```python
from build123d import *

# Parameters (mm, degrees)
ESQUISSE1_W                                        = 100
ESQUISSE1_H                                        = 50
BOSS_EXTRU_1_DEPTH                                 = 10
ESQUISSE2_W                                        = 100
ESQUISSE2_H                                        = 8
BOSS_EXTRU_2_DEPTH                                 = 30
ESQUISSE3_W                                        = 10
ESQUISSE3_H                                        = 34
BOSS_EXTRU_3_DEPTH                                 = 30
ESQUISSE5_R                                        = 5.25
ENL_V_MAT_EXTRU_1_DEPTH                            = 111.566721937
ENL_V_MAT_EXTRU_4_DEPTH                            = 82.240384046
CHAMBRAGE_POUR_VIS_T_TE_RONDE_BOMB_E_M_D           = 5.5
CHAMBRAGE_POUR_VIS_T_TE_RONDE_BOMB_E_M_CBORE_D     = 10
CHAMBRAGE_POUR_VIS_T_TE_RONDE_BOMB_E_M_CBORE_DEPTH = 5


with BuildPart() as part:
    # Esquisse1 → Boss.-Extru.1 (new body)
    with BuildSketch(Plane(origin=(0, 0, 0), x_dir=(1, 0, 0), z_dir=(0, 1, 0))):
        Rectangle(ESQUISSE1_W, ESQUISSE1_H)
    extrude(amount=BOSS_EXTRU_1_DEPTH)

    # Esquisse2 → Boss.-Extru.2 (add)
    with BuildSketch(Plane(origin=(0, 10, 0), x_dir=(1, 0, 0), z_dir=(0, 1, 0))):
        with Locations((0, -21)):
            Rectangle(ESQUISSE2_W, ESQUISSE2_H)
        with Locations((0, 21)):
            Rectangle(ESQUISSE2_W, ESQUISSE2_H)
    extrude(amount=BOSS_EXTRU_2_DEPTH)

    # Esquisse3 → Boss.-Extru.3 (add)
    with BuildSketch(Plane(origin=(0, 10, 0), x_dir=(1, 0, 0), z_dir=(0, 1, 0))):
        with Locations((-45, 0)):
            Rectangle(ESQUISSE3_W, ESQUISSE3_H)
    extrude(amount=BOSS_EXTRU_3_DEPTH)

    # Esquisse5 → Enlèv. mat.-Extru.1 (cut, through all)
    with BuildSketch(Plane.ZY.offset(50)):
        with Locations((0, 25)):
            Circle(ESQUISSE5_R)
    extrude(amount=-ENL_V_MAT_EXTRU_1_DEPTH, mode=Mode.SUBTRACT)

    # Esquisse8 → Enlèv. mat.-Extru.4 (cut, through all)
    with BuildSketch(Plane.XY.offset(25)):
        with BuildLine():
            Line((-20, 28.5), (40, 28.5))
            ThreePointArc((40, 28.5), (43.5, 25), (40, 21.5))
            Line((40, 21.5), (-20, 21.5))
            ThreePointArc((-20, 21.5), (-23.5, 25), (-20, 28.5))
        make_face()
    extrude(amount=-ENL_V_MAT_EXTRU_4_DEPTH, mode=Mode.SUBTRACT)

    # Chambrage pour vis à tête ronde bombée M51 (through all)
    with Locations(Plane(origin=(0, 10, 0), x_dir=(1, 0, 0), z_dir=(0, 1, 0))):
        with Locations((-25, 0), (0, 0)):
            CounterBoreHole(CHAMBRAGE_POUR_VIS_T_TE_RONDE_BOMB_E_M_D / 2, CHAMBRAGE_POUR_VIS_T_TE_RONDE_BOMB_E_M_CBORE_D / 2, CHAMBRAGE_POUR_VIS_T_TE_RONDE_BOMB_E_M_CBORE_DEPTH)


solid = part.part
```
Input: part model. Units: mm. Frame: model coordinates. A direction names the side the tool comes from. Coordinates: 2 decimals unless noted, no trailing zeros. Loops run counter-clockwise (first coordinate to the right, second up) from the corner with the lowest first, then second, coordinate; pieces in that order, holes last. Notation, with made-up numbers: (25.5, 34.25) - (61.5, 34.25) arc R29 ccw to (61.5, 54.25) - close; hole circle Ø1 at (39, 86). An arc over 180 degrees is marked (long way). Answer in a Markdown table with one row per item.
(1) Cut plane B-B on x = 0. Output: boundary loops of the cut face in (y, z).
Model answer:
| item | result |
|---|---|
| outline | (0, -25) - (21.5, -25) - (21.5, -17) - (10, -17) - (10, -5) - (5, -5) - (5, -2.75) - (0, -2.75) - close; (0, 2.75) - (5, 2.75) - (5, 5) - (10, 5) - (10, 17) - (21.5, 17) - (21.5, 25) - (0, 25) - close; (28.5, -25) - (40, -25) - (40, -17) - (28.5, -17) - close; (28.5, 17) - (40, 17) - (40, 25) - (28.5, 25) - close |
(2) Material intervals for L1, parallel to Y at x = -45.5, z = 0; L2, parallel to Y at x = 22, z = 18; L3, parallel to Z at x = 5, y = 29.5, sorted ascending. Write a range as from..to.
Model answer:
| item | result |
|---|---|
| L1 | y = 0..19.75, 30.25..40 |
| L2 | y = 0..21.5, 28.5..40 |
| L3 | z = -25..-17, 17..25 |
(3) Set-up query: faces 5 (the face through (2.2, 5, 2.2)), 6 (the face through (4, 21, 17)), 7 (the face through (10, 28.5, -21)). Return all of +Z, -Z, +X, -X, +Y, -Y with unobstructed straight access to the full face (end or side cutting, diameter ignored); none if empty.
Model answer:
| item | result |
|---|---|
| face 5 | +Y |
| face 6 | +X, +Y |
| face 7 | +Z, -Z |
(4) Mould query, pull axis X, two halves, no side actions, for faces 1 (the face through (-45.07, 20.34, 2.42)), 2 (the face through (50, 6, 6)), 3 (the face through (-23.5, 24.9, 21.1)), 4 (the face through (10, 28.5, 21)). Classes: pulls with the +X half, pulls with the -X half, needs draft (parallel to the pull), parting line crosses it, or undercut.
Model answer:
| item | result |
|---|---|
| face 1 | needs draft |
| face 2 | pulls with the +X half |
| face 3 | undercut |
| face 4 | undercut |
(5) Cut plane C-C on y = 25. Output: boundary loops of the cut face in (x, z), plus the area to 3 significant figures.
Model answer:
| item | result |
|---|---|
| outline | (-50, -25) - (-23.5, -25) - (-23.5, -17) - (-40, -17) - (-40, -5.25) - (-50, -5.25) - close; (-50, 5.25) - (-40, 5.25) - (-40, 17) - (-23.5, 17) - (-23.5, 25) - (-50, 25) - close; (43.5, -25) - (50, -25) - (50, -17) - (43.5, -17) - close; (43.5, 17) - (50, 17) - (50, 25) - (43.5, 25) - close |
| area | 763 mm² |
(6) Pin query (flat end, axial travel): P1, Ø9, axis at x = 14, z = 20.5, coming from the -Y side; P2, Ø11, axis at x = -1, z = 2.5, coming from the +Y side; P3, Ø6, axis at x = -25, z = 0, coming from the +Y side. Return the tip coordinate at first contact, or that it passes through.
Model answer:
| item | result |
|---|---|
| P1 | stops at y = 0 |
| P2 | stops at y = 10 |
| P3 | stops at y = 5 |
(7) Cut plane D-D on x = 21. Output: boundary loops of the cut face in (y, z).
Model answer:
| item | result |
|---|---|
| outline | (0, -25) - (21.5, -25) - (21.5, -17) - (10, -17) - (10, 17) - (21.5, 17) - (21.5, 25) - (0, 25) - close; (28.5, -25) - (40, -25) - (40, -17) - (28.5, -17) - close; (28.5, 17) - (40, 17) - (40, 25) - (28.5, 25) - close |
(8) Cut plane A-A on z = 0. Output: boundary loops of the cut face in (x, y).
Model answer:
| item | result |
|---|---|
| outline | (-50, 0) - (-27.75, 0) - (-27.75, 5) - (-30, 5) - (-30, 10) - (-40, 10) - (-40, 19.75) - (-50, 19.75) - close; (-50, 30.25) - (-40, 30.25) - (-40, 40) - (-50, 40) - close; (-22.25, 0) - (-2.75, 0) - (-2.75, 5) - (-5, 5) - (-5, 10) - (-20, 10) - (-20, 5) - (-22.25, 5) - close; (2.75, 0) - (50, 0) - (50, 10) - (5, 10) - (5, 5) - (2.75, 5) - close |
